```python
from build123d import *

# Parameters (mm, degrees)
SKETCH1_W               = 150
SKETCH1_H               = 170
BOSS_EXTRUDE1_DEPTH     = 10
CUT_EXTRUDE1_DEPTH      = 114.798066767
CUT_EXTRUDE1_DEPTH_BACK = 114.798066767
SKETCH4_R               = 4
SKETCH4_R_2             = 5
SKETCH4_W               = 10
SKETCH4_H               = 100
FILLET1_R               = 5
FILLET2_R               = 10


with BuildPart() as part:
    # Sketch1 → Boss-Extrude1 (new body)
    with BuildSketch(Plane(origin=(0, 0, 0), x_dir=(0, 0, -1), z_dir=(1, 0, 0))):
        Rectangle(SKETCH1_W, SKETCH1_H)
    extrude(amount=BOSS_EXTRUDE1_DEPTH)

    # Sketch4 → Cut-Extrude1 (cut, two sides: drawn at the far end of the back side and taken through both)
    with BuildSketch(Plane.ZY.offset(-CUT_EXTRUDE1_DEPTH_BACK)):
        with Locations((-60, 70)):
            Circle(SKETCH4_R)
        with Locations((0, 70)):
            Circle(SKETCH4_R)
        with Locations((60, 70)):
            Circle(SKETCH4_R)
        with Locations((0, 25)):
            Circle(SKETCH4_R_2)
        with BuildLine():
            Line((-40, -85), (40, -85))
            ThreePointArc((40, -85), (36.464466094, -83.535533906), (35, -80))
            Line((35, -80), (35, -30))
            ThreePointArc((35, -30), (33.535533906, -26.464466094), (30, -25))
            Line((30, -25), (-30, -25))
            ThreePointArc((-30, -25), (-33.535533906, -26.464466094), (-35, -30))
            Line((-35, -30), (-35, -80))
            ThreePointArc((-35, -80), (-36.464466094, -83.535533906), (-40, -85))
        make_face()
        with Locations((60, -20)):
            Rectangle(SKETCH4_W, SKETCH4_H)
        with Locations((-60, -20)):
            Rectangle(SKETCH4_W, SKETCH4_H)
    extrude(amount=CUT_EXTRUDE1_DEPTH + CUT_EXTRUDE1_DEPTH_BACK, mode=Mode.SUBTRACT)

    # Fillet1
    fillet1_edges = [part.edges().sort_by_distance(p)[0] for p in [
        (5, 30, 55),
        (5, 30, 65),
        (5, -70, 65),
        (5, -70, 55),
        (5, 30, -65),
        (5, 30, -55),
        (5, -70, -55),
        (5, -70, -65),
    ]]
    fillet(fillet1_edges, radius=FILLET1_R - 0.0001)  # a hair under: the kernel refuses the full size

    # Fillet2
    fillet2_edges = [part.edges().sort_by_distance(p)[0] for p in [
        (5, -85, -75),
        (5, -85, 75),
        (5, 85, 75),
        (5, 85, -75),
    ]]
    fillet(fillet2_edges, radius=FILLET2_R)


solid = part.part
```
For this review, take the finished solid that the model builds, in its own axes (mm). A direction names the side the tool comes from. Coordinates: 2 decimals unless noted, no trailing zeros. Order: outer loops, then holes, each group sorted by start corner. A loop starts at its lowest first (then second) coordinate and runs counter-clockwise, first axis right, second up. Notation, with made-up numbers: (-32, 11.25) - (-1, 11.25) arc R36 ccw to (-1, 45.25) - close; hole circle Ø4 at (10.5, 72.25). An arc over 180 degrees is marked (long way). Answer as a JSON object with one key per item and string values. Group by question number.
1. We need section A-A on z = 0. State the section outline as (x, y) points, then the cut area to 3 significant figures.
2. The part is to be moulded in two halves that separate along Y. For faces 4 (the cylindrical face through (5.07, -81.99, -72.15)), 5 (the cylindrical face through (5.07, 82.15, -71.99)), 6 (the cylindrical face through (5, -68, -56)), say which applies: pulls with the +Y half, pulls with the -Y half, needs draft (parallel to the pull), parting line crosses it, or undercut.
3. For faces 1 (the cylindrical face through (5.07, -81.99, 72.15)), 2 (the cylindrical face through (5, -26, -33)), 3 (the flat face through (5, -21, -65)), list the 3-axis set-ups (+Z, -Z, +X, -X, +Y, -Y) from which the entire face can be reached by the end or side of a thin tool; tool diameter is ignored.
4. For probe 1 along Z at (x, y) = (3.5, -19.5); probe 2 along Y at (x, z) = (2.5, -60); probe 3 along Z at (x, y) = (4.25, 70), list the stretches that pass through material, from the lowest coordinate up.
5. Clearance check with flat-ended pins moving along their axes: P1, Ø5, axis at x = 4, z = -10, coming from the -Y side; P2, Ø4, axis at x = 8.5, z = -32.5, coming from the -Y side. State where each tip first meets the part, or that it passes through.
6. We need section B-B on y = 70. State the section outline as (x, z) points.
7. We need section D-D on x = 8.25. Give the number of separate pieces and of enclosed holes in the cut face, then the cut area to 3 significant figures.
8. We need section C-C on y = -33. State the section outline as (x, z) points, then the cut area to 3 significant figures.
Final values:
{
 "1": {"outline": "(0, -25) - (10, -25) - (10, 20) - (0, 20) - close; (0, 30) - (10, 30) - (10, 66) - (0, 66) - close; (0, 74) - (10, 74) - (10, 85) - (0, 85) - close", "area": "920 mm²"},
 "2": {"face 4": "pulls with the -Y half", "face 5": "pulls with the +Y half", "face 6": "undercut"},
 "3": {"face 1": "+Z, +X, -X, -Y", "face 2": "+X, -X, -Y", "face 3": "+X, -X"},
 "4": {"probe 1": "-75 to -65, -55 to 55, 65 to 75", "probe 2": "-85 to -70, 30 to 66, 74 to 85", "probe 3": "-75 to -64, -56 to -4, 4 to 56, 64 to 75"},
 "5": {"P1": "y = -25", "P2": "y = -27.82"},
 "6": {"outline": "(0, -75) - (10, -75) - (10, -64) - (0, -64) - close; (0, -56) - (10, -56) - (10, -4) - (0, -4) - close; (0, 4) - (10, 4) - (10, 56) - (0, 56) - close; (0, 64) - (10, 64) - (10, 75) - (0, 75) - close"},
 "7": {"separate pieces": "1", "enclosed holes": "6", "area": "19,000 mm²"},
 "8": {"outline": "(0, -75) - (10, -75) - (10, -65) - (0, -65) - close; (0, -55) - (10, -55) - (10, -35) - (0, -35) - close; (0, 35) - (10, 35) - (10, 55) - (0, 55) - close; (0, 65) - (10, 65) - (10, 75) - (0, 75) - close", "area": "600 mm²"}
}
